Source: CAD feature listing. Evaluate the final solid. Frame: model axes, mm. A direction names the side the tool comes from. Round coordinates to 2 decimals unless told otherwise and drop trailing zeros. Write item = value, one per line.
from build123d import *

# Parameters (mm, degrees)
SKETCH16_R                = 3.3274
SKETCH16_R_2              = 2.5527
F_15_1575_PROFILE_1_DEPTH = 290


with BuildPart() as part:
    # Sketch16 → 15 1575 PROFILE(1) (new body)
    with BuildSketch(Plane.XZ.offset(-145)):
        with BuildLine():
            Line((-9.398, 5.461), (-5.334, 5.461))
            ThreePointArc((-5.334, 5.461), (-4.435974388, 5.832974388), (-4.064, 6.731))
            Line((-4.064, 6.731), (-4.064, 8.001))
            ThreePointArc((-4.064, 8.001), (-4.510369265, 9.078630735), (-5.588, 9.525))
            Line((-5.588, 9.525), (-15.875, 9.525))
            ThreePointArc((-15.875, 9.525), (-18.12006403, 8.59506403), (-19.05, 6.35))
            Line((-19.05, 6.35), (-19.05, -6.35))
            ThreePointArc((-19.05, -6.35), (-18.12006403, -8.59506403), (-15.875, -9.525))
            Line((-15.875, -9.525), (15.875, -9.525))
            ThreePointArc((15.875, -9.525), (18.12006403, -8.59506403), (19.05, -6.35))
            Line((19.05, -6.35), (19.05, 6.35))
            ThreePointArc((19.05, 6.35), (18.12006403, 8.59506403), (15.875, 9.525))
            Line((15.875, 9.525), (5.588, 9.525))
            ThreePointArc((5.588, 9.525), (4.510369265, 9.078630735), (4.064, 8.001))
            Line((4.064, 8.001), (4.064, 6.731))
            ThreePointArc((4.064, 6.731), (4.435974388, 5.832974388), (5.334, 5.461))
            Line((5.334, 5.461), (9.398, 5.461))
            ThreePointArc((9.398, 5.461), (10.026617928, 5.200617928), (10.287, 4.572))
            Line((10.287, 4.572), (10.287, 4.255364987))
            ThreePointArc((10.287, 4.255364987), (10.219328904, 3.915159416), (10.026617928, 3.626747059))
            Line((10.026617928, 3.626747059), (5.124055081, -1.275815789))
            ThreePointArc((5.124055081, -1.275815789), (3.583109058, -2.305443004), (1.765439291, -2.667))
            Line((1.765439291, -2.667), (-1.765439291, -2.667))
            ThreePointArc((-1.765439291, -2.667), (-3.583109058, -2.305443004), (-5.124055081, -1.275815789))
            Line((-5.124055081, -1.275815789), (-10.026617928, 3.626747059))
            ThreePointArc((-10.026617928, 3.626747059), (-10.219328904, 3.915159416), (-10.287, 4.255364987))
            Line((-10.287, 4.255364987), (-10.287, 4.572))
            ThreePointArc((-10.287, 4.572), (-10.026617928, 5.200617928), (-9.398, 5.461))
        make_face()
        with Locations((-12.7, -3.175)):
            Circle(SKETCH16_R, mode=Mode.SUBTRACT)
        with Locations((-14.848796959, 5.276432773)):
            Circle(SKETCH16_R_2, mode=Mode.SUBTRACT)
        with Locations((12.7, -3.175)):
            Circle(SKETCH16_R, mode=Mode.SUBTRACT)
        with Locations((14.848796959, 5.276432773)):
            Circle(SKETCH16_R_2, mode=Mode.SUBTRACT)
    extrude(amount=F_15_1575_PROFILE_1_DEPTH)


solid = part.part
1. Contact query for flat-ended pins moving along their axis: pin 1 Ø0.6 at (y, z) = (3, 7) entering from +X; pin 2 Ø3 at (x, y) = (0, -3) entering from +Z; pin 3 Ø0.6 at (y, z) = (19.5, 7.5) entering from -X. Output: stop coordinate, or through.
Evaluation:
pin_1 = 19.03
pin_2 = -2.67
pin_3 = -18.93
2. Line query: probe 1 along X at (y, z) = (133, -3.75); probe 2 along X at (y, z) = (46, -4); probe 3 along Z at (x, y) = (15, 66) (1 decimal). Output: solid intervals per line, ascending. Write a range as from..to.
Evaluation:
probe_1 = -19.05..-15.98, -9.42..9.42, 15.98..19.05
probe_2 = -19.05..-15.92, -9.48..9.48, 15.92..19.05
probe_3 = -9.5..-5.6, -0.8..2.7, 7.8..9.5
3. Mould query, pull axis X, two halves, no side actions, for faces 3 (the face through (-19.05, 2, 0)), 4 (the face through (11, 2, 9.525)), 5 (the face through (17.284, 2.03, 6.043)). Classes: released by +X, released by -X, zero draft, split by the parting line, or undercut.
Evaluation:
face_3 = released by -X
face_4 = zero draft
face_5 = undercut
4. Section query A-A (y = 73). Give the number of separate pieces and of enclosed holes in the cut face, then the cut area to 3 significant figures.
Evaluation:
separate_pieces = 1
enclosed_holes = 4
area = 449 mm²
5. Set-up query: faces 1 (the face through (-11, 2, 9.525)), 2 (the face through (7.6, 2, 1.2)). Return all of +Z, -Z, +X, -X, +Y, -Y with unobstructed straight access to the full face (end or side cutting, diameter ignored); none if empty.
Evaluation:
face_1 = +Z, +X, -X, +Y, -Y
face_2 = +Y, -Y
